For this review, take the finished solid that the model builds, in its own axes (mm). Face numbers are marked on the shaded views. A direction names the side the tool comes from. Round coordinates to 2 decimals unless told otherwise and drop trailing zeros. Write each loop counter-clockwise with the first axis right and the second up, starting at its lowest first coordinate (ties: lowest second). Pieces come first, ordered by that corner, then holes. Notation, with made-up numbers: (45, 5) - (95, 5) arc R27 ccw to (95, 39) - close; hole circle Ø2 at (36, 1). An arc over 180 degrees is marked (long way). One line per item, written item: value. Start each with the question number.
Q1. Mouldability with a two-part tool opening along Z and no side actions: class the marked faces 1, 2 and 3 as +Z half, -Z half, draft (parallel to the pull), parting line (faces both ways), or undercut.
Q2. Add section A-A on x = 0. Write out the cut boundary in (y, z).
Q3. Add section B-B on z = 0. Write out the cut boundary in (x, y), and give its area (4 significant figures).
Q4. Add section C-C on y = 22.75. Write out the cut boundary in (x, z), and give its area (3 significant figures).
Q5. Add section D-D on x = 11.5. Write out the cut boundary in (y, z).
Q6. Clearance check with flat-ended pins moving along their axes: pin 1 Ø1.5 at (y, z) = (24.5, 12.5) entering from +X; pin 2 Ø5 at (x, z) = (1.5, 15.5) entering from +Y; pin 3 Ø3 at (y, z) = (17, 16) entering from -X; pin 4 Ø5 at (x, y) = (-9, 3.5) entering from +Z. State where each tip first meets the part, or that it passes through.
Q7. Tool access review of the marked faces 4 and 5: name each direction out of +Z, -Z, +X, -X, +Y, -Y from which nothing blocks a thin tool from reaching the whole face with its end or side.
Q8. For probe 1 along X at (y, z) = (11.75, 0); probe 2 along X at (y, z) = (18.75, 15); probe 3 along Z at (x, y) = (0.25, 2), list the stretches that pass through material, from the lowest coordinate up.
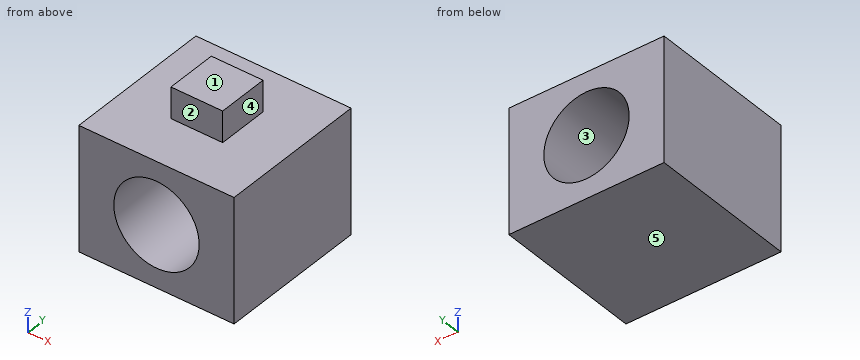
```python
from build123d import *

# Parameters (mm, degrees)
SKETCH1_W           = 30
SKETCH1_H           = 29
BOSS_EXTRUDE1_DEPTH = 12
SKETCH2_R           = 8.25
CUT_EXTRUDE1_DEPTH  = 34
BOSS_EXTRUDE2_START = 12
SKETCH3_W           = 10
SKETCH3_H           = 10
BOSS_EXTRUDE2_DEPTH = 6


with BuildPart() as part:
    # Sketch1 → Boss-Extrude1 (new, symmetric)
    with BuildSketch(Plane.XY):
        with Locations((0, 14.5)):
            Rectangle(SKETCH1_W, SKETCH1_H)
    extrude(amount=BOSS_EXTRUDE1_DEPTH, both=True)

    # Sketch2 → Cut-Extrude1 (cut, symmetric)
    with BuildSketch(Plane(origin=(0, 0, 0), x_dir=(1, 0, 0), z_dir=(0, 1, 0))):
        with Locations(Location((0, 0, 0), (0, 0, 270))):
            Circle(SKETCH2_R)
    extrude(amount=CUT_EXTRUDE1_DEPTH, both=True, mode=Mode.SUBTRACT)

    # Sketch3 → Boss-Extrude2 (add)
    with BuildSketch(Plane.XY.offset(BOSS_EXTRUDE2_START)):
        with Locations((0, 15)):
            Rectangle(SKETCH3_W, SKETCH3_H)
    extrude(amount=BOSS_EXTRUDE2_DEPTH)


solid = part.part
```
Result set:
1. face 1: +Z half
1. face 2: draft
1. face 3: undercut
2. outline: (0, -12) - (29, -12) - (29, -8.25) - (0, -8.25) - close; (0, 8.25) - (29, 8.25) - (29, 12) - (20, 12) - (20, 18) - (10, 18) - (10, 12) - (0, 12) - close
3. outline: (-15, 0) - (-8.25, 0) - (-8.25, 29) - (-15, 29) - close; (8.25, 0) - (15, 0) - (15, 29) - (8.25, 29) - close
3. area: 391.5 mm^2
4. outline: (-15, -12) - (15, -12) - (15, 12) - (-15, 12) - close; hole circle Ø16.5 at (0, 0)
4. area: 506 mm^2
5. outline: (0, -12) - (29, -12) - (29, 12) - (0, 12) - close
6. pin 1: stops at x = 15
6. pin 2: stops at y = 20
6. pin 3: stops at x = -5
6. pin 4: stops at z = 12
7. face 4: +Z, +X, +Y, -Y
7. face 5: -Z, +X, -X, +Y, -Y
8. probe 1: x = -15 to -8.25, 8.25 to 15
8. probe 2: x = -5 to 5
8. probe 3: z = -12 to -8.25, 8.25 to 12
